Model file for the job. Use its own axes, mm. A direction names the side the tool comes from. Give positions to 0.01 mm unless a question says otherwise; leave off trailing zeros. Loops run counter-clockwise (first coordinate to the right, second up) from the corner with the lowest first, then second, coordinate; pieces in that order, holes last. Notation, with made-up numbers: M -4,24 L 41,24 A20 cw 41,60 Z; hole C 39.25,-20.5 d11. An arc over 180 degrees is marked long. Use CSV: the item, a comma, the result in double quotes. Start each with the question number.
(1) Slice it at C-C on y = 12.5. List the corners of the cut face in (x, z), and give its area (3 significant figures).
(2) Tool access for faces 4 (the face through (-23.87, 2.71, 5.57)), 5 (the face through (-22.35, 10.43, -6.48)): list every direction of +Z, -Z, +X, -X, +Y, -Y with a clear straight run to the whole face (end or side of a thin tool).
(3) Slice it at B-B on y = 2.5. List the corners of the cut face in (x, z), and give its area (3 significant figures).
(4) Two-plate mould, pull along X, no slides. Class faces 1 (the face through (-30, 8, 12)), 2 (the face through (-27.693, 8, -9)), 3 (the face through (-23.87, 2.71, -10.43)): pulls with the +X half, pulls with the -X half, needs draft (parallel to the pull), parting line crosses it, or undercut.
(5) Wall check: line 1 along Z through (x, y) = (-23, 2); line 2 along Z through (x, y) = (-24.25, 5); line 3 along Y through (x, z) = (-18, 6.5). Give the ranges that are in metal, low to high. Write a range as from..to.
(6) Flat gauge pins, fed straight in: P1, Ø4, axis at x = -19.5, z = 7.5, coming from the -Y side; P2, Ø2, axis at x = -30.5, y = 11, coming from the -Z side; P3, Ø8, axis at y = 10, z = -15.5, coming from the -X side. Where does each tip first touch, or does it go through?
(7) Slice it at A-A on z = 8. List the corners of the cut face in (x, y), and give its area (3 significant figures).
(8) Slice it at D-D on x = -17.25. List the corners of the cut face in (y, z), and give its area (3 significant figures).
```python
from build123d import *

# Parameters (mm, degrees)
F0_R     = 4
F0_R_2   = 2.25
F0_W     = 1
F0_H     = 20
F1_DEPTH = 15.5
F2_DEPTH = 15.501
F3_DEPTH = 5.5


with BuildPart() as f1:
    # F0 (on Front) → F1 (new body)
    with BuildSketch(Plane.XZ):
        with BuildLine():
            Line((-31.693068, 12), (-27.693068, 12))
            Line((-27.693068, 12), (-27.693068, -10))
            Line((-27.693068, -10), (-26.693068, -10))
            Line((-26.693068, -10), (-26.693068, -30))
            Line((-26.693068, -30), (-22.693068, -30))
            Line((-22.693068, -30), (-22.693068, -18))
            ThreePointArc((-22.693068, -18), (-21.228602, -14.464466), (-17.693068, -13))
            Line((-17.693068, -13), (-13.693068, -13))
            Line((-13.693068, -13), (-13.693068, 30))
            Line((-13.693068, 30), (-31.693068, 30))
            Line((-31.693068, 30), (-31.693068, 12))
        make_face()
        with Locations((-20.693068, -8)):
            Circle(F0_R, mode=Mode.SUBTRACT)
        with Locations((-20.693068, 8)):
            Circle(F0_R, mode=Mode.SUBTRACT)
        with Locations((-20.693068, 8)):
            Circle(F0_R)
        with Locations((-20.693068, 8)):
            Circle(F0_R_2, mode=Mode.SUBTRACT)
        with Locations((-20.693068, -8)):
            Circle(F0_R)
        with Locations((-20.693068, -8)):
            Circle(F0_R_2, mode=Mode.SUBTRACT)
        with BuildLine():
            Line((-22.693068, -18), (-22.693068, -30))
            Line((-22.693068, -30), (-13.693068, -30))
            Line((-13.693068, -30), (-13.693068, -13))
            Line((-13.693068, -13), (-17.693068, -13))
            ThreePointArc((-17.693068, -13), (-21.228602, -14.464466), (-22.693068, -18))
        make_face()
        with Locations((-20.693068, 8)):
            Circle(F0_R_2)
        with Locations((-27.193068, -20)):
            Rectangle(F0_W, F0_H)
        with Locations((-20.693068, -8)):
            Circle(F0_R_2)
    extrude(amount=-F1_DEPTH)

    # F0 (on Front) → F2 (cut, through all)
    with BuildSketch(Plane.XZ):
        with Locations((-20.693068, 8)):
            Circle(F0_R_2)
        with Locations((-20.693068, -8)):
            Circle(F0_R_2)
    extrude(amount=-F2_DEPTH, mode=Mode.SUBTRACT)

    # F0 (on Front) → F3 (cut)
    with BuildSketch(Plane.XZ):
        with Locations((-20.693068, 8)):
            Circle(F0_R)
        with Locations((-20.693068, 8)):
            Circle(F0_R_2, mode=Mode.SUBTRACT)
        with Locations((-20.693068, -8)):
            Circle(F0_R)
        with Locations((-20.693068, -8)):
            Circle(F0_R_2, mode=Mode.SUBTRACT)
        with Locations((-20.693068, 8)):
            Circle(F0_R_2)
        with Locations((-20.693068, -8)):
            Circle(F0_R_2)
    extrude(amount=-F3_DEPTH, mode=Mode.SUBTRACT)


solid = f1.part
```
Reply:
1,outline,"M -31.69,12 L -27.69,12 L -27.69,-30 L -13.69,-30 L -13.69,30 L -31.69,30 Z; hole C -20.69,-8 d4.5; hole C -20.69,8 d4.5"
1,area,"880 mm^2"
2,face 4,"-Y"
2,face 5,"+Y, -Y"
3,outline,"M -31.69,12 L -27.69,12 L -27.69,-30 L -13.69,-30 L -13.69,30 L -31.69,30 Z; hole C -20.69,-8 d8; hole C -20.69,8 d8"
3,area,"811 mm^2"
4,face 1,"needs draft"
4,face 2,"pulls with the -X half"
4,face 3,"undercut"
5,line 1,"z = -30..-11.27, -4.73..4.73, 11.27..30"
5,line 2,"z = -30..-9.83, -6.17..6.17, 9.83..30"
5,line 3,"y = 5.5..15.5"
6,P1,"stops at y = 5.5"
6,P2,"stops at z = 12"
6,P3,"stops at x = -27.69"
7,outline,"M -27.69,0 L -24.69,0 L -24.69,5.5 L -22.94,5.5 L -22.94,15.5 L -27.69,15.5 Z; M -18.44,5.5 L -16.69,5.5 L -16.69,0 L -13.69,0 L -13.69,15.5 L -18.44,15.5 Z"
7,area,"128 mm^2"
8,outline,"M 0,-30 L 15.5,-30 L 15.5,30 L 0,30 L 0,10.04 L 5.5,10.04 L 5.5,5.96 L 0,5.96 L 0,-5.96 L 5.5,-5.96 L 5.5,-10.04 L 0,-10.04 Z"
8,area,"885 mm^2"
